Geometry check sheet. Reference: the model listing, model coordinates, mm. A direction names the side the tool comes from. Give positions to 0.01 mm unless a question says otherwise; leave off trailing zeros. Write each loop counter-clockwise with the first axis right and the second up, starting at its lowest first coordinate (ties: lowest second). Pieces come first, ordered by that corner, then holes. Notation, with made-up numbers: (-9.5, 24) - (5.5, 24) arc R18 cw to (5.5, 55) - close; hole circle Ø10 at (43, 9). An arc over 180 degrees is marked (long way). Write item = value, one per line. Start each with the question number.
(1) Draft check along Y on faces 1 (the flat face through (59.142, 47, 0)), 2 (the flat face through (0, 26, 0)), 3 (the flat face through (44.78, 44.49, 0.09)). Enter one of: pulls with the +Y half, pulls with the -Y half, needs draft (parallel to the pull), parting line crosses it, or undercut.
(2) Access from +Z, -Z, +X, -X, +Y, -Y to the whole of each face (thin tool, end or side, straight path). Record for faces 4 (the flat face through (0, 13, -11.85)), 5 (the flat face through (15, 15, 0)), 6 (the flat face through (48, 41, 6.1)).
(3) Section check A-A, the plane y = 14. Enter the section's corners in (x, z), plus the area to 3 significant figures.
(4) Section check C-C, the plane x = -2. Enter the section's corners in (y, z).
(5) Depth check by flat-ended pin: pin 1 Ø1.3 at (x, y) = (51.46, 43.54) entering from +Z; pin 2 Ø15 at (y, z) = (20.5, -1) entering from +X; pin 3 Ø12 at (x, z) = (-5, 4.5) entering from -Y. Enter the tip coordinate at first touch or a pass-through.
(6) Section check B-B, the plane z = -5.25. Enter the section's corners in (x, y), plus the area to 3 significant figures.
(7) Thickness scan on L1, parallel to Z at x = -5, y = 6; L2, parallel to Z at x = 50, y = 44.5. Record the ranges inside material, lowest first.
(8) Section check D-D, the plane z = -9. Enter the section's corners in (x, y), plus the area to 3 significant figures.
```python
from build123d import *

# Parameters (mm, degrees)
BOSS_EXTRUDE1_DEPTH = 15
SKETCH2_W           = 23.7
SKETCH2_H           = 23.7
CUT_EXTRUDE1_DEPTH  = 26
SKETCH5_W           = 12.2
SKETCH5_H           = 12.2
CUT_EXTRUDE3_DEPTH  = 10.4
SKETCH6_R           = 1.1
CUT_EXTRUDE4_DEPTH  = 84.052948209
SKETCH7_R           = 1.1
CUT_EXTRUDE5_DEPTH  = 84.052948209


with BuildPart() as part:
    # Sketch1 → Boss-Extrude1 (new, symmetric)
    with BuildSketch(Plane.XY):
        Polygon((0, 0), (15, 0), (15, 30), (45, 30), (59.142135624, 44.142135624), (59.142135624, 50), (-15, 50), (-15, 0), align=None)
    extrude(amount=BOSS_EXTRUDE1_DEPTH, both=True)

    # Sketch2 → Cut-Extrude1 (cut)
    with BuildSketch(Plane.XZ):
        Rectangle(SKETCH2_W, SKETCH2_H)
    extrude(amount=-CUT_EXTRUDE1_DEPTH, mode=Mode.SUBTRACT)

    # Sketch5 → Cut-Extrude3 (cut)
    with BuildSketch(Plane(origin=(7.5, -7.5, 0), x_dir=(0, 0, -1), z_dir=(0.7071067811865487, -0.7071067811865465, 0))):
        with Locations((0, 63.033008589)):
            Rectangle(SKETCH5_W, SKETCH5_H)
    extrude(amount=-CUT_EXTRUDE3_DEPTH, mode=Mode.SUBTRACT)

    # Sketch6 → Cut-Extrude4 (cut, through all)
    with BuildSketch(Plane.XY.offset(15)):
        with Locations((51.46, 43.54)):
            Circle(SKETCH6_R)
    extrude(amount=-CUT_EXTRUDE4_DEPTH, mode=Mode.SUBTRACT)

    # Sketch7 → Cut-Extrude5 (cut, through all)
    with BuildSketch(Plane.XY.offset(15)):
        with Locations((46.714373567, 38.394222143)):
            Circle(SKETCH7_R)
    extrude(amount=-CUT_EXTRUDE5_DEPTH, mode=Mode.SUBTRACT)


solid = part.part
```
Model answer:
q1.face_1 = needs draft
q1.face_2 = pulls with the -Y half
q1.face_3 = undercut
q2.face_4 = -Y
q2.face_5 = +Z, -Z, +X, -Y
q2.face_6 = none
q3.outline = (-15, -15) - (15, -15) - (15, 15) - (-15, 15) - close; hole (-11.85, -11.85) - (11.85, -11.85) - (11.85, 11.85) - (-11.85, 11.85) - close
q3.area = 338 mm²
q4.outline = (0, -15) - (50, -15) - (50, 15) - (0, 15) - (0, 11.85) - (26, 11.85) - (26, -11.85) - (0, -11.85) - close
q5.pin_1 = through
q5.pin_2 = 15
q5.pin_3 = 26
q6.outline = (-15, 0) - (-11.85, 0) - (-11.85, 26) - (11.85, 26) - (11.85, 0) - (15, 0) - (15, 30) - (45, 30) - (47.76, 32.76) - (40.4, 40.11) - (49.03, 48.74) - (56.38, 41.38) - (59.14, 44.14) - (59.14, 50) - (-15, 50) - close
q6.area = 1,540 mm²
q7.L1 = -15 to -11.85, 11.85 to 15
q7.L2 = -15 to -6.1, 6.1 to 15
q8.outline = (-15, 0) - (-11.85, 0) - (-11.85, 26) - (11.85, 26) - (11.85, 0) - (15, 0) - (15, 30) - (45, 30) - (59.14, 44.14) - (59.14, 50) - (-15, 50) - close; hole circle Ø2.2 at (46.71, 38.39); hole circle Ø2.2 at (51.46, 43.54)
q8.area = 1,660 mm²
